Answer from the drawing. Dimensions are ordinates in mm from the lowest x, y and z of the part. A direction names the side the tool comes from. Give positions to 0.01 mm unless a question says otherwise; leave off trailing zeros. Loops run counter-clockwise (first coordinate to the right, second up) from the corner with the lowest first, then second, coordinate; pieces in that order, holes last.
(1) Which of the six approach directions +Z, -Z, +X, -X, +Y, -Y give full straight-line access (tool end or side, diameter ignored) to the marked faces 1 and 2?
(2) Determine the mould class of the marked faces 3, 4, 5 and 6 for opening direction Z: pulls with the +Z half, pulls with the -Z half, needs draft (parallel to the pull), parting line crosses it, or undercut.
(3) Find section B-B, the plane y = 20.5. State how many separate pieces and enclosed holes the cut face has, then the cut area to 3 significant figures.
(4) Find section A-A, the plane x = 127. Write down the section's boundary in (y, z), then the cut area to 3 significant figures.
(5) This flat-tipped pin is pushed along its axis until it touches: P1, Ø19, axis at y = 24, z = 30.5, coming from the -X side. Where does it stop, or does it pass through?
(6) Find section D-D, the plane x = 25.4. Write down the section's boundary in (y, z) (3 decimals).
(7) Straight lines are drawn through the part: probe 1 along Z at (x, y) = (41, 24.5); probe 2 along Y at (x, z) = (25.4, 46) (3 decimals); probe 3 along X at (y, z) = (19, 46) (1 decimal). For each, find the intervals that lie inside material, in ascending order.
(8) Find section C-C, the plane z = 28. Write down the section's boundary in (x, y) (1 decimal).
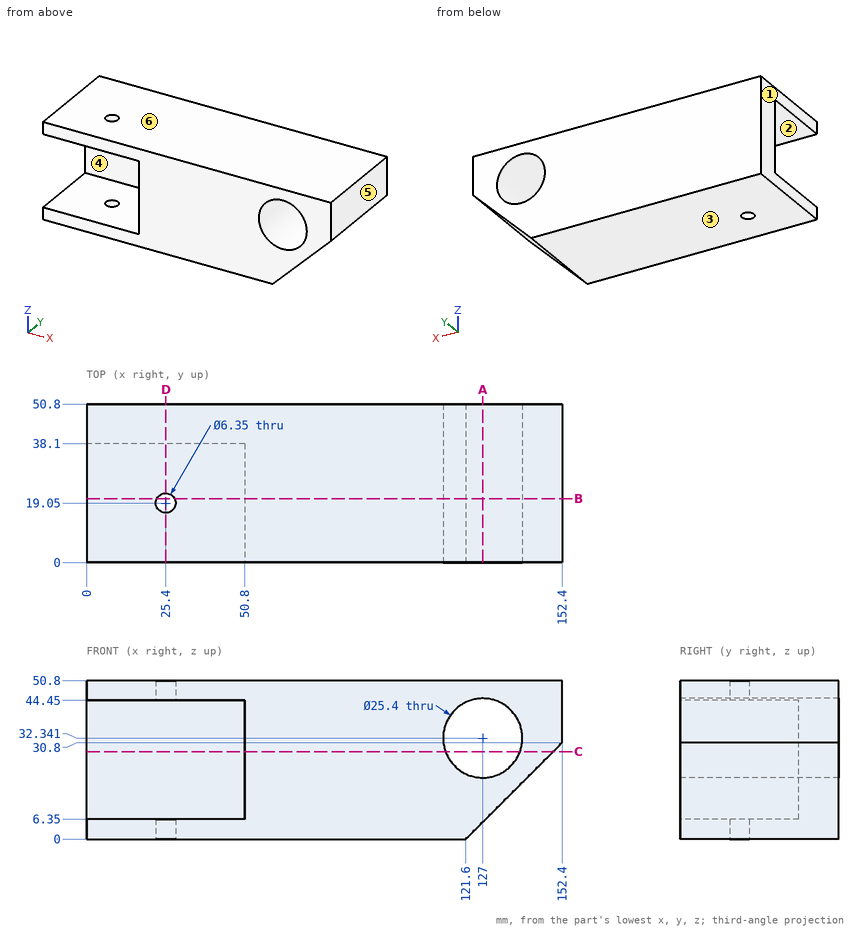
Entries:
1. face 1: +Z, -Z, -X, +Y, -Y
1. face 2: -X, -Y
2. face 3: pulls with the -Z half
2. face 4: undercut
2. face 5: needs draft
2. face 6: pulls with the +Z half
3. separate pieces: 3
3. enclosed holes: 1
3. area: 4,750 mm2
4. outline: (0, 5.4) - (50.8, 5.4) - (50.8, 19.64) - (0, 19.64) - close; (0, 45.04) - (50.8, 45.04) - (50.8, 50.8) - (0, 50.8) - close
4. area: 1,020 mm2
5. P1: stops at x = 50.8
6. outline: (0, 0) - (15.875, 0) - (15.875, 6.35) - (0, 6.35) - close; (0, 44.45) - (15.875, 44.45) - (15.875, 50.8) - (0, 50.8) - close; (22.225, 0) - (50.8, 0) - (50.8, 50.8) - (22.225, 50.8) - (22.225, 44.45) - (38.1, 44.45) - (38.1, 6.35) - (22.225, 6.35) - close
7. probe 1: z = 0 to 6.35, 44.45 to 50.8
7. probe 2: y = 0 to 15.875, 22.225 to 50.8
7. probe 3: x = 0 to 22.2, 28.6 to 152.4
8. outline: (0, 38.1) - (50.8, 38.1) - (50.8, 0) - (115.1, 0) - (115.1, 50.8) - (0, 50.8) - close; (138.9, 0) - (149.6, 0) - (149.6, 50.8) - (138.9, 50.8) - close
